from build123d import *


with BuildPart() as part:
    # Esquisse1 → Révolution1 (revolve)
    with BuildSketch(Plane(origin=(0, 0, 0), x_dir=(0, 0, -1), z_dir=(1, 0, 0))):
        with BuildLine():
            Line((10.5, 0), (3, 0))
            ThreePointArc((3, 0), (2.121320344, -2.121320344), (0, -3))
            Line((0, -3), (0, 0))
            Line((0, 0), (0, 20))
            Line((0, 20), (0, 22))
            Line((0, 22), (5, 22))
            Line((5, 22), (5, 20))
            Line((5, 20), (10, 20))
            Line((10, 20), (10, 1))
            Line((10, 1), (10.5, 1))
            Line((10.5, 1), (10.5, 0))
        make_face()
    revolve(axis=Axis((0, 0, 0), (0, 1, 0)))


solid = part.part
Input: part model. Units: mm. Frame: model coordinates. A direction names the side the tool comes from. Coordinates: 2 decimals unless noted, no trailing zeros. Order: outer loops, then holes, each group sorted by start corner. A loop starts at its lowest first (then second) coordinate and runs counter-clockwise, first axis right, second up. Notation, with made-up numbers: M -20,75.25 L 3,75.25 A27 ccw 3,96.25 Z; hole C 2,-29.75 d6. An arc over 180 degrees is marked long. Answer as CSV lines item,"result".
1. Section B-B (x = 0). Return the cut outline in (y, z).
Reported:
outline,"M 0,-10.5 L 1,-10.5 L 1,-10 L 20,-10 L 20,-5 L 22,-5 L 22,5 L 20,5 L 20,10 L 1,10 L 1,10.5 L 0,10.5 L 0,3 A3 ccw 0,-3 Z"
2. Section A-A (z = 0). Return the cut outline in (x, y).
Reported:
outline,"M -10.5,0 L -3,0 A3 ccw 3,0 L 10.5,0 L 10.5,1 L 10,1 L 10,20 L 5,20 L 5,22 L -5,22 L -5,20 L -10,20 L -10,1 L -10.5,1 Z"
3. Material intervals for line 1 (Y direction, x = 6.75, z = -2.25); line 2 (Y direction, x = -3.75, z = -0.5); line 3 (Z direction, x = -4.75, y = 16), sorted ascending. Write a range as from..to.
Reported:
line 1,"0..20"
line 2,"0..22"
line 3,"-8.8..8.8"
4. Section D-D (x = 8.5). Return the cut outline in (y, z).
Reported:
outline,"M 0,-6.16 L 1,-6.16 L 1,-5.27 L 20,-5.27 L 20,5.27 L 1,5.27 L 1,6.16 L 0,6.16 Z"
5. Access query for faces 1 (the cylindrical face through (-3.2, 0.5, -10)), 2 (the flat face through (-2.5, 0, -2.2)), 3 (the cylindrical face through (4.88, 20.99, 1.08)). Directions: +Z, -Z, +X, -X, +Y, -Y. A direction counts if a zero-diameter tool reaches every point of the face in a straight line with its end or side. Return the directions, or none.
Reported:
face 1,"+Y, -Y"
face 2,"-Y"
face 3,"+Y"
6. First-contact query: P1, Ø3, axis at x = -6.5, y = 19, coming from the -Z side; P2, Ø12, axis at y = 7.5, z = -1.5, coming from the +X side; P3, Ø1.5, axis at x = 3.5, z = -6, coming from the +Y side; P4, Ø12, axis at x = 3, z = 3, coming from the -Y side. Flat tips, straight axial feed; report the tip coordinate or a pass-through.
Reported:
P1,"z = -8.66"
P2,"x = 10"
P3,"y = 20"
P4,"y = -3"
7. Section C-C (y = 9.5). Return the cut outline in (x, z).
Reported:
outline,"C 0,0 d20"
